```python
from build123d import *

# Parameters (mm, degrees)
F1_DEPTH = 40.2336
F0_R     = 10.16
F2_DEPTH = 15.7734
F3_R     = 3.302


with BuildPart() as f1:
    # F0 (on Top) → F1 (new body)
    with BuildSketch(Plane.XY):
        with BuildLine():
            ThreePointArc((27.2897645342, 23.8900197129), (28.2518640674, 28.0782870201), (28.575, 32.3634709971))
            ThreePointArc((28.575, 32.3634709971), (-4.2851839771, 60.6153350645), (-27.2897645342, 23.8900197129))
            ThreePointArc((-27.2897645342, 23.8900197129), (0, 3.7884709971), (27.2897645342, 23.8900197129))
        make_face()
        with BuildLine():
            ThreePointArc((-4.5638517477, 18.8244934333), (-8.3344653219, 43.9681831455), (14.2875, 32.3634709971))
            ThreePointArc((14.2875, 32.3634709971), (11.7649813941, 24.2568151486), (5.0881482523, 19.0126881133))
            Line((5.0881482523, 19.0126881133), (5.0881482523, 13.8341709971))
            Line((5.0881482523, 13.8341709971), (-4.5638517477, 13.8341709971))
            Line((-4.5638517477, 13.8341709971), (-4.5638517477, 18.8244934333))
        make_face(mode=Mode.SUBTRACT)
    extrude(amount=F1_DEPTH)

    # F0 (on Top) → F2 (join)
    with BuildSketch(Plane.XY):
        with BuildLine():
            ThreePointArc((27.2897645342, 23.8900197129), (0, 3.7884709971), (-27.2897645342, 23.8900197129))
            Line((-27.2897645342, 23.8900197129), (-19.0398767625, -20.990567758))
            ThreePointArc((-19.0398767625, -20.990567758), (0, -2.5615290029), (19.0398767625, -20.990567758))
            Line((19.0398767625, -20.990567758), (27.2897645342, 23.8900197129))
        make_face()
        with BuildLine():
            ThreePointArc((19.0398767625, -20.990567758), (0, -2.5615290029), (-19.0398767625, -20.990567758))
            Line((-19.0398767625, -20.990567758), (-17.5744174222, -28.9628793733))
            ThreePointArc((-17.5744174222, -28.9628793733), (0, -40.6615290029), (17.5744174222, -28.9628793733))
            Line((17.5744174222, -28.9628793733), (19.0398767625, -20.990567758))
        make_face()
        with Locations((0, -21.6115290029)):
            Circle(F0_R, mode=Mode.SUBTRACT)
    extrude(amount=F2_DEPTH)

    # F3
    f3_edges = [f1.edges().sort_by_distance(p)[0] for p in [
        (27.289765, 40.836922, 40.2336),
    ]]
    fillet(f3_edges, radius=F3_R)


solid = f1.part
```
Model file for the job. Use its own axes, mm. A direction names the side the tool comes from. Give positions to 0.01 mm unless a question says otherwise; leave off trailing zeros. Order: outer loops, then holes, each group sorted by start corner. A loop starts at its lowest first (then second) coordinate and runs counter-clockwise, first axis right, second up.
1) Mould opens along Y. For faces 1 (the flat face through (0, 11, 0)), 2 (the flat face through (22.364, -2.906, 7.776)), 3 (the cylindrical face through (-1.323, -11.538, 7.776)) say: +Y half, -Y half, draft (parallel to the pull), parting line (faces both ways), or undercut.
2) Pin check, flat tips, straight feed: pin 1 (6 mm diameter, centred on y = 25, z = 34, fed in from +X); pin 2 (4 mm diameter, centred on y = 16.5, z = 26.5, fed in from -X); pin 3 (23 mm diameter, centred on x = 0, y = 32.36, fed in from -Z); pin 4 (1 mm diameter, centred on x = -14.5, z = 5.5, fed in from -Y). Stop position of each tip, or through.
3) 3-axis set-ups, long thin cutter, end or side, ignore diameter. For faces 4 (the flat face through (-4.564, 16, 20)), 5 (the cylindrical face through (-0.31, -40.66, 7.78)): which of +Z, -Z, +X, -X, +Y, -Y reach the whole face in a straight line?
4) Saw through at B-B, the plane y = -16. Write the cut outline in (x, z).
5) Saw through at C-C, the plane z = 7. Count the separate pieces of the cut face and the enclosed holes in it, then the cut area to 3 significant figures.
6) Wall check: probe 1 along Y at (x, z) = (0, 8); probe 2 along Y at (x, z) = (0, 30); probe 3 along Z at (x, y) = (16.5, -28.5). Give the ranges that are in metal, low to high.
Computed:
1. face 1: draft
1. face 2: -Y half
1. face 3: undercut
2. pin 1: stops at x = 28.24
2. pin 2: stops at x = -24.99
2. pin 3: passes through
2. pin 4: stops at y = -34.53
3. face 4: +Z, -Z
3. face 5: +Z, -Z, -Y
4. outline: (-19.96, 0) - (-8.47, 0) - (-8.47, 15.77) - (-19.96, 15.77) - close; (8.47, 0) - (19.96, 0) - (19.96, 15.77) - (8.47, 15.77) - close
5. separate pieces: 1
5. enclosed holes: 2
5. area: 3,420 mm2
6. probe 1: y = -40.66 to -31.77, -11.45 to 13.83, 46.65 to 60.94
6. probe 2: y = 3.79 to 13.83, 46.65 to 60.94
6. probe 3: z = 0 to 15.77
